from build123d import *

# Parameters (mm, degrees)
F1_DEPTH        = 5
F2_DEPTH        = 5
F2_COPIES_COUNT = 11
F2_COPIES_ANGLE = 150
F3_R            = 12.5
F4_DEPTH        = 10.001


# Not quite as in the source:
# - a pattern or mirror of a feature is missing from the dataset's text; its kind, count and spacing are read off the source's solid


with BuildPart() as f1:
    # F0 (on Front) → F1 (new body, symmetric)
    with BuildSketch(Plane.XZ):
        with BuildLine():
            Line((-25.0008701164, 31.2242933215), (-63.4987428752, 0.3995663471))
            ThreePointArc((-63.4987428752, 0.3995663471), (-59.9818720369, -20.842865133), (-49.5685656478, -39.6888813097))
            Line((-49.5685656478, -39.6888813097), (0, 0))
            Line((0, 0), (-25.0008701164, 31.2242933215))
        make_face()
        with BuildLine():
            Line((0, 0), (62.772077735, 9.5872966381))
            ThreePointArc((62.772077735, 9.5872966381), (-4.6082108818, 63.3325697605), (-63.4987428752, 0.3995663471))
            Line((-63.4987428752, 0.3995663471), (-25.0008701164, 31.2242933215))
            Line((-25.0008701164, 31.2242933215), (0, 0))
        make_face()
        with BuildLine():
            ThreePointArc((-39.3237135407, -49.8587560351), (27.705542678, -57.1371412036), (63.5, 0))
            ThreePointArc((63.5, 0), (63.3177579206, 4.8074454664), (62.772077735, 9.5872966381))
            Line((62.772077735, 9.5872966381), (0, 0))
            Line((0, 0), (-49.5685656478, -39.6888813097))
            ThreePointArc((-49.5685656478, -39.6888813097), (-44.7360694833, -45.065886069), (-39.3237135407, -49.8587560351))
        make_face()
        with BuildLine():
            ThreePointArc((-49.5685656478, -39.6888813097), (-59.9818720369, -20.842865133), (-63.4987428752, 0.3995663471))
            Line((-63.4987428752, 0.3995663471), (-727.5474698493, -531.2952842967))
            Line((-727.5474698493, -531.2952842967), (-702.5465997329, -562.5195776181))
            Line((-702.5465997329, -562.5195776181), (-49.5685656478, -39.6888813097))
        make_face()
    extrude(amount=F1_DEPTH, both=True)

    # F0 (on Front) → F2 (join, symmetric)
    with BuildSketch(Plane.XZ):
        with BuildLine():
            Line((-53.9442142409, -56.1162132047), (-39.3237135407, -49.8587560351))
            ThreePointArc((-39.3237135407, -49.8587560351), (-44.7360694833, -45.065886069), (-49.5685656478, -39.6888813097))
            Line((-49.5685656478, -39.6888813097), (-55.718461724, -54.3549506266))
            Line((-55.718461724, -54.3549506266), (-53.9442142409, -56.1162132047))
        make_face()
    f2 = extrude(amount=F2_DEPTH, both=True)

    # F2_copies: F2 ×11 about axis
    f2_copies_axis = Axis((0, 0, 0), (0, -1, 0))
    for i in range(1, F2_COPIES_COUNT):
        add(f2.rotate(f2_copies_axis, i * F2_COPIES_ANGLE / (F2_COPIES_COUNT - 1)))

    # F3 (on face) → F4 (cut, through all)
    with BuildSketch(Plane(origin=(0, 5, 0), x_dir=(-1, 0, 0), z_dir=(0, 1, 0))):
        Circle(F3_R)
    extrude(amount=-F4_DEPTH, mode=Mode.SUBTRACT)


solid = f1.part
Work out the finished part from the listing and answer in its coordinate system (mm). Give positions to 0.01 mm unless a question says otherwise; leave off trailing zeros. Write each loop counter-clockwise with the first axis right and the second up, starting at its lowest first coordinate (ties: lowest second). Pieces come first, ordered by that corner, then holes.
Q1. The part is cut by section A-A on z = -331. Give the vertices of the cut face in (x, y).
Answer:
outline: (-477.39, -5) - (-413.4, -5) - (-413.4, 5) - (-477.39, 5) - close
Q2. Given pin 1 (6 mm diameter, centred on x = -517, y = 1.5, fed in from +Z); pin 2 (4 mm diameter, centred on y = -3, z = -432, fed in from -X); pin 3 (1.5 mm diameter, centred on x = -124.5, y = 4, fed in from +Z), each flat-ended and moving along its own axis, determine where each tip first touches the part or whether it passes through.
Answer:
pin 1: stops at z = -360.31
pin 2: stops at x = -606.03
pin 3: stops at z = -47.84
Q3. Straight lines are drawn through the part: L1, parallel to Z at x = 0, y = 2; L2, parallel to Z at x = -241, y = -2.75; L3, parallel to Z at x = -380.5, y = 1.25. For each, find the intervals that lie inside material, in ascending order.
Answer:
L1: z = -77.83 to -12.5, 12.5 to 63.5
L2: z = -192.97 to -141.72
L3: z = -304.66 to -253.42
Q4. For a pull along Z with two mould halves and no side action, classify faces 1 (the face through (-11.923, 0.07, 3.755)), 2 (the face through (-390.875, -0.07, -261.726)), 3 (the face through (-715.22, -0.07, -546.69)), 4 (the face through (-285, 5, -208)) as released by +Z, released by -Z, zero draft, split by the parting line, or undercut.
Answer:
face 1: undercut
face 2: released by +Z
face 3: released by -Z
face 4: zero draft
Q5. The part is cut by section B-B on x = -379. Give the vertices of the cut face in (y, z), and give its area (3 significant figures).
Answer:
outline: (-5, -303.46) - (5, -303.46) - (5, -252.22) - (-5, -252.22) - close
area: 512 mm2
